```python
from build123d import *

# Parameters (mm, degrees)
F0_R     = 0.325
F0_W     = 0.54
F0_H     = 1.2
F1_DEPTH = 2.5


with BuildPart() as f1:
    # F0 (on Top) → F1 (new body)
    with BuildSketch(Plane.XY):
        Polygon((-71.271986, 0), (-69.271986, 0), (-69.271986, 0.4), (-69.271986, 1.6), (-69.271986, 2), (-71.271986, 2), align=None)
        with Locations((-70.271986, 1)):
            Circle(F0_R, mode=Mode.SUBTRACT)
        with Locations((-69.001986, 1)):
            Rectangle(F0_W, F0_H)
        Polygon((-68.731986, 1.6), (-68.731986, 0.4), (-68.731986, 0), (-66.731986, 0), (-66.731986, 0.4), (-66.731986, 1.6), (-66.731986, 2), (-68.731986, 2), align=None)
        with Locations((-67.731986, 1)):
            Circle(F0_R, mode=Mode.SUBTRACT)
        with Locations((-66.461986, 1)):
            Rectangle(F0_W, F0_H)
        Polygon((-66.191986, 1.6), (-66.191986, 0.4), (-66.191986, 0), (-64.191986, 0), (-64.191986, 0.4), (-64.191986, 1.6), (-64.191986, 2), (-66.191986, 2), align=None)
        with Locations((-65.191986, 1)):
            Circle(F0_R, mode=Mode.SUBTRACT)
        with Locations((-63.921986, 1)):
            Rectangle(F0_W, F0_H)
        Polygon((-63.651986, 1.6), (-63.651986, 0.4), (-63.651986, 0), (-61.651986, 0), (-61.651986, 0.4), (-61.651986, 1.6), (-61.651986, 2), (-63.651986, 2), align=None)
        with Locations((-62.651986, 1)):
            Circle(F0_R, mode=Mode.SUBTRACT)
        with Locations((-61.381986, 1)):
            Rectangle(F0_W, F0_H)
        Polygon((-61.111986, 1.6), (-61.111986, 0.4), (-61.111986, 0), (-59.111986, 0), (-59.111986, 0.4), (-59.111986, 1.6), (-59.111986, 2), (-61.111986, 2), align=None)
        with Locations((-60.111986, 1)):
            Circle(F0_R, mode=Mode.SUBTRACT)
        with Locations((-58.841986, 1)):
            Rectangle(F0_W, F0_H)
        Polygon((-58.571986, 1.6), (-58.571986, 0.4), (-58.571986, 0), (-56.571986, 0), (-56.571986, 0.4), (-56.571986, 1.6), (-56.571986, 2), (-58.571986, 2), align=None)
        with Locations((-57.571986, 1)):
            Circle(F0_R, mode=Mode.SUBTRACT)
        with Locations((-56.301986, 1)):
            Rectangle(F0_W, F0_H)
        Polygon((-56.031986, 1.6), (-56.031986, 0.4), (-56.031986, 0), (-54.031986, 0), (-54.031986, 0.4), (-54.031986, 1.6), (-54.031986, 2), (-56.031986, 2), align=None)
        with Locations((-55.031986, 1)):
            Circle(F0_R, mode=Mode.SUBTRACT)
        with Locations((-53.761986, 1)):
            Rectangle(F0_W, F0_H)
        Polygon((-53.491986, 1.6), (-53.491986, 0.4), (-53.491986, 0), (-51.491986, 0), (-51.491986, 0.4), (-51.491986, 1.6), (-51.491986, 2), (-53.491986, 2), align=None)
        with Locations((-52.491986, 1)):
            Circle(F0_R, mode=Mode.SUBTRACT)
        with Locations((-51.221986, 1)):
            Rectangle(F0_W, F0_H)
        Polygon((-50.951986, 1.6), (-50.951986, 0.4), (-50.951986, 0), (-48.951986, 0), (-48.951986, 0.4), (-48.951986, 1.6), (-48.951986, 2), (-50.951986, 2), align=None)
        with Locations((-49.951986, 1)):
            Circle(F0_R, mode=Mode.SUBTRACT)
        with Locations((-48.681986, 1)):
            Rectangle(F0_W, F0_H)
        Polygon((-48.411986, 1.6), (-48.411986, 0.4), (-48.411986, 0), (-46.411986, 0), (-46.411986, 0.4), (-46.411986, 1.6), (-46.411986, 2), (-48.411986, 2), align=None)
        with Locations((-47.411986, 1)):
            Circle(F0_R, mode=Mode.SUBTRACT)
        with Locations((-46.141986, 1)):
            Rectangle(F0_W, F0_H)
        Polygon((-45.871986, 1.6), (-45.871986, 0.4), (-45.871986, 0), (-43.871986, 0), (-43.871986, 0.4), (-43.871986, 1.6), (-43.871986, 2), (-45.871986, 2), align=None)
        with Locations((-44.871986, 1)):
            Circle(F0_R, mode=Mode.SUBTRACT)
        with Locations((-43.601986, 1)):
            Rectangle(F0_W, F0_H)
        Polygon((-43.331986, 1.6), (-43.331986, 0.4), (-43.331986, 0), (-41.331986, 0), (-41.331986, 0.4), (-41.331986, 1.6), (-41.331986, 2), (-43.331986, 2), align=None)
        with Locations((-42.331986, 1)):
            Circle(F0_R, mode=Mode.SUBTRACT)
        with Locations((-41.061986, 1)):
            Rectangle(F0_W, F0_H)
        Polygon((-40.791986, 1.6), (-40.791986, 0.4), (-40.791986, 0), (-38.791986, 0), (-38.791986, 0.4), (-38.791986, 1.6), (-38.791986, 2), (-40.791986, 2), align=None)
        with Locations((-39.791986, 1)):
            Circle(F0_R, mode=Mode.SUBTRACT)
        with Locations((-38.521986, 1)):
            Rectangle(F0_W, F0_H)
        Polygon((-38.251986, 1.6), (-38.251986, 0.4), (-38.251986, 0), (-36.251986, 0), (-36.251986, 0.4), (-36.251986, 1.6), (-36.251986, 2), (-38.251986, 2), align=None)
        with Locations((-37.251986, 1)):
            Circle(F0_R, mode=Mode.SUBTRACT)
    extrude(amount=F1_DEPTH)


solid = f1.part
```
Build history of the part. All positions in model axes, mm. Give positions to 0.01 mm unless a question says otherwise; leave off trailing zeros. Use a Markdown table: item, result.
(1) Drop a flat-ended pin along its axis: pin 1 Ø1.5 at (x, z) = (-63, 2) entering from -Y. Give the stop position or say it passes through.
Taken from the geometry:
| item | result |
|---|---|
| pin 1 | y = 0 |
(2) Band-saw the part on A-A (z = 2.1). Give the number of separate pieces and of enclosed holes in the cut face, and give its area (3 significant figures).
Taken from the geometry:
| item | result |
|---|---|
| separate pieces | 1 |
| enclosed holes | 14 |
| area | 59.8 mm2 |
(3) Wall check: line 1 along Y through (x, z) = (-38.5, 2.25); line 2 along Y through (x, z) = (-67.5, 0.95); line 3 along Y through (x, z) = (-60, 1.45). Give the ranges that are in metal, low to high.
Taken from the geometry:
| item | result |
|---|---|
| line 1 | 0.4 to 1.6 |
| line 2 | 0 to 0.77, 1.23 to 2 |
| line 3 | 0 to 0.69, 1.31 to 2 |
